Autodesk Inventor part; units mm, degrees
ref_plane "YZ Plane" through (0, 0, 0) normal (1, 0, 0) x (0, 1, 0)
ref_plane "XZ Plane" through (0, 0, 0) normal (0, 1, 0) x (-1, 0, 0)
ref_plane "XY Plane" through (0, 0, 0) normal (0, 0, 1) x (1, 0, 0)
sketch "Sketch1" plane through (0, 0, 0) normal (0, 0, 1) x (1, 0, 0)
  line L0 (-5.08, 8.636) -> (5.08, 8.636)
  line L1 (5.08, 8.636) -> (5.08, 0)
  line L2 (5.08, 0) -> (-5.08, 0)
  line L3 (-5.08, 0) -> (-5.08, 8.636)
  point P0 (0, 0)
  point P1 (0, 0)
  dimension "d0" = 10.16
  dimension "d1" = 8.636
extrude "Extrusion1" add sketch "Sketch1" along normal blind 4.4704
sketch "Sketch2" plane through (-5.08, 8.636, 0) normal (0, 1, 0) x (1, 0, 0)
  line L0 (0.0889, -1.397) -> (10.0711, -1.397)
  line L1 (10.0711, -1.397) -> (10.0711, 0)
  line L2 (10.0711, 0) -> (0.0889, 0)
  line L3 (0.0889, 0) -> (0.0889, -1.397)
  line L4 (0, 0) -> (10.16, 0)
  point P0 (5.08, 0)
  dimension "d7" = 1.397
  dimension "d8" = 9.9822
extrude "Extrusion2" add sketch "Sketch2" along normal blind 6.35
sketch "Sketch3" plane through (-4.9911, 8.636, 1.397) normal (0, 0, 1) x (1, 0, 0)
  line L0 (9.9822, 6.35) -> (0, 6.35)
  line L1 (9.9822, 0) -> (9.9822, 6.35)
  line L2 (4.9911, 6.35) -> (4.9911, 1.588) construction
  point P0 (4.9911, 3.81)
  dimension "d9" = 2.54
hole "Hole1" at (0, 12.446, 1.397) direction (0, 0, -1) diameter 3.683 end through all
sketch "Sketch4" plane through (-5.08, 0, 0) normal (0, -1, 0) x (1, 0, 0)
  line L0 (0, 0) -> (0, 4.4704)
  line L1 (10.16, 0) -> (10.16, 4.4704)
  line L2 (0, 2.2352) -> (10.16, 2.2352) construction
  line L3 (1.905, 2.5273) -> (3.175, 2.5273)
  line L4 (3.175, 2.5273) -> (3.175, 1.9431)
  line L5 (3.175, 1.9431) -> (1.905, 1.9431)
  line L6 (1.905, 1.9431) -> (1.905, 2.5273)
  point P0 (1.905, 2.2352)
  dimension "d17" = 0.5842
  dimension "d18" = 1.27
  dimension "d19" = 1.905
extrude "Extrusion3" add sketch "Sketch4" along normal blind 3.81
sketch "Sketch5" plane through (-5.08, -3.81, 0) normal (0, -1, 0) x (1, 0, 0)
  line L0 (1.905, 2.5273) -> (3.175, 2.5273)
  line L1 (3.175, 1.9431) -> (1.905, 1.9431)
  line L2 (2.1336, 2.5273) -> (2.9464, 2.5273)
  line L3 (2.9464, 2.5273) -> (2.9464, 1.9431)
  line L4 (2.9464, 1.9431) -> (2.1336, 1.9431)
  line L5 (2.1336, 1.9431) -> (2.1336, 2.5273)
  point P0 (2.54, 1.9431)
  dimension "d22" = 0.8128
extrude "Extrusion4" add sketch "Sketch5" along normal blind 3.81
pattern_linear "Rectangular Pattern1" count 3 spacing 2.54 along (1, 0, 0) of "Extrusion4", "Extrusion3"
properties part number "Fet"
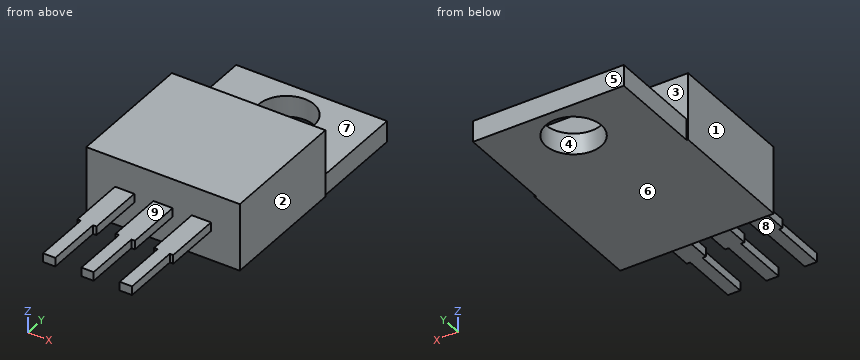
Source: CAD feature listing. Evaluate the final solid. Frame: model axes, mm. Face numbers are marked on the shaded views. A direction names the side the tool comes from. Give positions to 0.01 mm unless a question says otherwise; leave off trailing zeros. Order: outer loops, then holes, each group sorted by start corner. A loop starts at its lowest first (then second) coordinate and runs counter-clockwise, first axis right, second up.
(1) Section query C-C (z = 3.9). Return the cut outline in (x, y).
(2) Contact query for flat-ended pins moving along their axis: P1, Ø2, axis at x = 3, y = -5, coming from the -Z side; P2, Ø0.5, axis at y = -6.5, z = 2.5, coming from the +X side; P3, Ø0.6, axis at y = -6, z = 2, coming from the -X side. Output: stop coordinate, or through.
(3) Section query A-A (x = 0). Return the cut outline in (y, z), plus the area to 3 significant figures.
(4) Section query B-B (z = 2.3). Return the cut outline in (x, y) (3 decimals), plus the area to 3 significant figures.
(5) Material intervals for line 1 along Y through (x, z) = (0, 0.45); line 2 along Z through (x, y) = (0.75, 9); line 3 along Y through (x, z) = (-2, 1.3), sorted ascending.
(6) Access query for the marked faces 5, 6, 7, 8 and 9. Directions: +Z, -Z, +X, -X, +Y, -Y. A direction counts if a zero-diameter tool reaches every point of the face in a straight line with its end or side. Return the directions, or none.
(7) Pull-direction query (X, two-part tool) for the marked faces 1, 2, 3 and 4; classes: +X half, -X half, draft (parallel to the pull), parting line (faces both ways), or undercut.
Outcome:
1. outline: (-5.08, 0) - (5.08, 0) - (5.08, 8.64) - (-5.08, 8.64) - close
2. P1: stops at z = 1.94
2. P2: stops at x = 2.95
2. P3: stops at x = -2.95
3. outline: (-7.62, 1.94) - (0, 1.94) - (0, 0) - (10.6, 0) - (10.6, 1.4) - (8.64, 1.4) - (8.64, 4.47) - (0, 4.47) - (0, 2.53) - (-7.62, 2.53) - close; (14.29, 0) - (14.99, 0) - (14.99, 1.4) - (14.29, 1.4) - close
3. area: 46.8 mm2
4. outline: (-5.08, 0) - (-3.175, 0) - (-3.175, -3.81) - (-2.946, -3.81) - (-2.946, -7.62) - (-2.134, -7.62) - (-2.134, -3.81) - (-1.905, -3.81) - (-1.905, 0) - (-0.635, 0) - (-0.635, -3.81) - (-0.406, -3.81) - (-0.406, -7.62) - (0.406, -7.62) - (0.406, -3.81) - (0.635, -3.81) - (0.635, 0) - (1.905, 0) - (1.905, -3.81) - (2.134, -3.81) - (2.134, -7.62) - (2.946, -7.62) - (2.946, -3.81) - (3.175, -3.81) - (3.175, 0) - (5.08, 0) - (5.08, 8.636) - (-5.08, 8.636) - close
4. area: 112 mm2
5. line 1: y = 0 to 10.6, 14.29 to 14.99
5. line 2: z = 0 to 1.4
5. line 3: y = 0 to 14.99
6. face 5: +Z, -Z, +X, -X, +Y
6. face 6: -Z, +X, -X, +Y, -Y
6. face 7: +Z, +X, -X, +Y
6. face 8: -Z, +X, -X, -Y
6. face 9: +Z, +X, -X, -Y
7. face 1: -X half
7. face 2: +X half
7. face 3: draft
7. face 4: undercut
